Check sheet for the modelled part. Datum: model origin and axes. Units: mm. A direction names the side the tool comes from. Coordinates: 2 decimals unless noted, no trailing zeros. Order: outer loops, then holes, each group sorted by start corner. A loop starts at its lowest first (then second) coordinate and runs counter-clockwise, first axis right, second up.
from build123d import *

# Parameters (mm, degrees)
FILLET1_R              = 3
M4_TAPPED_HOLE1_REACH  = 34.296
M4_TAPPED_HOLE1_BORE_R = 1.65
CIRPATTERN1_COUNT      = 3


with BuildPart() as part:
    # Sketch1 → Revolve1 (revolve)
    with BuildSketch(Plane.XY, mode=Mode.PRIVATE) as revolve1_sk:
        Polygon((0, 0), (15, 0), (15, 5), (8, 5), (8, 17), (4, 17), (4, 5), (0, 5), align=None)
    revolve(revolve1_sk.sketch.rotate(Axis((0, 0, 0), (0, 1, 0)), 90), axis=Axis((0, 0, 0), (0, 1, 0)))

    # Fillet1
    fillet1_edges = [part.edges().sort_by_distance(p)[0] for p in [
        (0, 5, 8),
    ]]
    fillet(fillet1_edges, radius=FILLET1_R)

    # M4 Tapped Hole1 bore → M4 Tapped Hole1 (cut, up to next)
    with BuildSketch(Plane.XY.offset(8), mode=Mode.PRIVATE) as m4_tapped_hole1_sk1:
        with Locations((0, 12)):
            Circle(M4_TAPPED_HOLE1_BORE_R)
    m4_tapped_hole1_tool1 = extrude(m4_tapped_hole1_sk1.sketch, amount=-M4_TAPPED_HOLE1_REACH, mode=Mode.PRIVATE) & part.part
    m4_tapped_hole1 = m4_tapped_hole1_tool1.solids().sort_by_distance((0, 12, 8))[0]
    add(m4_tapped_hole1, mode=Mode.SUBTRACT)

    # CirPattern1: M4 Tapped Hole1 ×3 about axis
    cirpattern1_axis = Axis((0, 17, 0), (0, -1, 0))
    for i in range(1, CIRPATTERN1_COUNT):
        add(m4_tapped_hole1.rotate(cirpattern1_axis, i * 360 / CIRPATTERN1_COUNT), mode=Mode.SUBTRACT)


solid = part.part
(1) Thickness scan on probe 1 along Y at (x, z) = (0, 5.95); probe 2 along X at (y, z) = (10.5, 0); probe 3 along X at (y, z) = (12, 5.8). Record the ranges inside material, lowest first.
Filled in:
probe 1: y = 0 to 10.35, 13.65 to 17
probe 2: x = -8 to -4, 4 to 8
probe 3: x = -5.51 to -1.65, 1.65 to 5.51
(2) Cross-section at A-A (x = 0). Enter the section's corners in (y, z), and give its area (3 significant figures).
Filled in:
outline: (0, -15) - (5, -15) - (5, -11) arc R3 cw to (8, -8) - (17, -8) - (17, -4) - (5, -4) - (5, 4) - (10.35, 4) - (10.35, 8) - (8, 8) arc R3 cw to (5, 11) - (5, 15) - (0, 15) - close; (13.65, 4) - (17, 4) - (17, 8) - (13.65, 8) - close
area: 237 mm2
(3) Cross-section at B-B (z = 0). Enter the section's corners in (x, y).
Filled in:
outline: (-15, 0) - (15, 0) - (15, 5) - (11, 5) arc R3 cw to (8, 8) - (8, 17) - (4, 17) - (4, 5) - (-4, 5) - (-4, 17) - (-8, 17) - (-8, 8) arc R3 cw to (-11, 5) - (-15, 5) - close
(4) Cross-section at C-C (y = 12). Enter the section's corners in (x, z), and give its area (3 significant figures).
Filled in:
outline: (-7.6, -2.49) - (-3.98, -0.39) arc R4 cw to (-1.65, 3.64) - (-1.65, 7.83) arc R8 ccw to start; (-5.95, -5.34) arc R8 ccw to (5.95, -5.34) - (2.33, -3.25) arc R4 cw to (-2.33, -3.25) - close; (1.65, 3.64) arc R4 cw to (3.98, -0.39) - (7.6, -2.49) arc R8 ccw to (1.65, 7.83) - close
area: 111 mm2
(5) Tool access check on faces 4 (the cylindrical face through (-0.215, 13.636, 5.853)), 5 (the cylindrical face through (3.905, 10.916, 0.867)), 6 (the flat face through (2, 17, 4)). Record the directions out of +Z, -Z, +X, -X, +Y, -Y that give a thin tool (end or side, any length) a straight path to the whole face; none if there is none.
Filled in:
face 4: +Z
face 5: +Y
face 6: +Z, -Z, +X, -X, +Y
(6) Release check for a two-part mould opening along Z. For faces 1 (the cylindrical face through (-4.961, 13.636, -3.112)), 2 (the flat face through (-10, 5, 5)), 3 (the cylindrical face through (-12.65, 2.54, -8.06)) record: +Z half, -Z half, draft (parallel to the pull), parting line (faces both ways), or undercut.
Filled in:
face 1: undercut
face 2: draft
face 3: parting line
(7) Go/stop test with flat-tipped pins: P1, Ø4, axis at x = -10.5, z = 6, coming from the +Y side; P2, Ø1.5, axis at x = 1, y = 11, coming from the +Z side; P3, Ø6, axis at x = 2, y = 9.5, coming from the +Z side. Record where each tip stops, or that it passes through.
Filled in:
P1: stops at y = 5.14
P2: stops at z = 7.98
P3: stops at z = 8.26
(8) Cross-section at D-D (y = 15.75). Enter the section's corners in (x, z).
Filled in:
outline: circle Ø16 at (0, 0); hole circle Ø8 at (0, 0)
